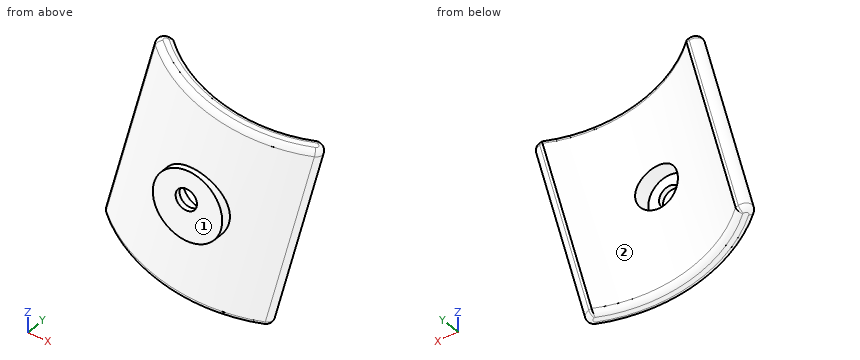
from build123d import *

# Parameters (mm, degrees)
CYLINDER016_R          = 8
CYLINDER016_DEPTH      = 10
CYLINDER016_ROLL_ANGLE = 90
CYLINDER015_R          = 4
CYLINDER015_DEPTH      = 20
CYLINDER015_ROLL_ANGLE = 90
BOX016_W               = 120
BOX016_H               = 100
BOX016_DEPTH           = 150
CYLINDER014_R          = 44
CYLINDER014_DEPTH      = 75
CYLINDER013_R          = 50
CYLINDER013_DEPTH      = 75
CYLINDER012_R          = 13
CYLINDER012_DEPTH      = 8
CYLINDER012_ROLL_ANGLE = 90
FILLET012_R            = 3
FILLET013_R            = 2
FILLET014_R            = 2
CUT021_PITCH_ANGLE     = 15


with BuildPart() as cylindre016:
    # Cylinder016 → Cylinder016 (new body)
    with BuildSketch(Plane.XY):
        Circle(CYLINDER016_R)
    extrude(amount=CYLINDER016_DEPTH)


with BuildPart() as cylindre016_1:
    # Cylinder016 roll: moved
    add(cylindre016.part.rotate(Axis((0, 0, 0), (1, 0, 0)), CYLINDER016_ROLL_ANGLE))


with BuildPart() as cylindre016_2:
    # Cylinder016 placement: moved
    add(cylindre016_1.part.moved(Location((-212, -9, -164))))


with BuildPart() as cylindre015:
    # Cylinder015 → Cylinder015 (new body)
    with BuildSketch(Plane.XY):
        Circle(CYLINDER015_R)
    extrude(amount=CYLINDER015_DEPTH)


with BuildPart() as cylindre015_1:
    # Cylinder015 roll: moved
    add(cylindre015.part.rotate(Axis((0, 0, 0), (1, 0, 0)), CYLINDER015_ROLL_ANGLE))


with BuildPart() as cylindre015_2:
    # Cylinder015 placement: moved
    add(cylindre015_1.part.moved(Location((-212, -10, -164))))


with BuildPart() as cube016:
    # Box016 → Box016 (new body)
    with BuildSketch(Plane(origin=(-269, -3, -220), x_dir=(1, 0, 0), z_dir=(0, 0, 1))):
        with Locations((60, 50)):
            Rectangle(BOX016_W, BOX016_H)
    extrude(amount=BOX016_DEPTH)


with BuildPart() as cylindre014:
    # Cylinder014 → Cylinder014 (new body)
    with BuildSketch(Plane(origin=(-212, 31, -203), x_dir=(1, 0, 0), z_dir=(0, 0, 1))):
        Circle(CYLINDER014_R)
    extrude(amount=CYLINDER014_DEPTH)


with BuildPart() as cut017:
    # Cylinder013 → Cylinder013 (new body)
    with BuildSketch(Plane(origin=(-212, 31, -203), x_dir=(1, 0, 0), z_dir=(0, 0, 1))):
        Circle(CYLINDER013_R)
    extrude(amount=CYLINDER013_DEPTH)

    # Cut017: cut Cylindre014
    add(cylindre014.part, mode=Mode.SUBTRACT)


with BuildPart() as cut021:
    # Cylinder012 → Cylinder012 (new body)
    with BuildSketch(Plane.XY):
        Circle(CYLINDER012_R)
    extrude(amount=CYLINDER012_DEPTH)


with BuildPart() as cut021_1:
    # Cylinder012 roll: moved
    add(cut021.part.rotate(Axis((0, 0, 0), (1, 0, 0)), CYLINDER012_ROLL_ANGLE))


with BuildPart() as cut021_2:
    # Cylinder012 placement: moved
    add(cut021_1.part.moved(Location((-211, -13, -166))))

    # Fusion011: union Cut017
    add(cut017.part)

    # Cut018: cut Cube016
    add(cube016.part, mode=Mode.SUBTRACT)

    # Fillet012
    fillet012_edges = [cut021_2.edges().sort_by_distance(p)[0] for p in [
        (-175.339394, -3, -165.5),
        (-248.660606, -3, -165.5),
    ]]
    fillet(fillet012_edges, radius=FILLET012_R)

    # Fillet013
    fillet013_edges = [cut021_2.edges().sort_by_distance(p)[0] for p in [
        (-212, -19, -203),
        (-212, -13, -203),
    ]]
    fillet(fillet013_edges, radius=FILLET013_R)

    # Fillet014
    fillet014_edges = [cut021_2.edges().sort_by_distance(p)[0] for p in [
        (-212, -19, -128),
        (-212, -13, -128),
    ]]
    fillet(fillet014_edges, radius=FILLET014_R)

    # Cut019: cut Cylindre015
    add(cylindre015_2.part, mode=Mode.SUBTRACT)

    # Cut021: cut Cylindre016
    add(cylindre016_2.part, mode=Mode.SUBTRACT)


with BuildPart() as cut021_3:
    # Cut021 pitch: moved
    add(cut021_2.part.rotate(Axis((0, 0, 0), (0, 1, 0)), CUT021_PITCH_ANGLE))


with BuildPart() as cut021_4:
    # Cut021 placement: moved
    add(cut021_3.part.moved(Location((35.610827, 0, -60.508913))))


solid = cut021_4.part
Can you work these out from the model? Positions are in its coordinate system, mm. Face numbers are marked on the shaded views. Give positions to 0.01 mm unless a question says otherwise; leave off trailing zeros. One line per item, written item: value.
1) I'm going to push flat-ended pins straight in: pin 1 (4 mm diameter, centred on y = -9, z = -163, fed in from +X); pin 2 (2 mm diameter, centred on x = -193.5, z = -190.5, fed in from +Y); pin 3 (4 mm diameter, centred on x = -232, y = -13, fed in from -Z). Where does each tip first touch, or does it pass through?
Geometry check:
pin 1: stops at x = -178.24
pin 2: stops at y = -4.97
pin 3: stops at z = -199.43
2) Thinking about a two-plate mould opening in X: for the marked faces 1 and 2, which applies, +X half, -X half, draft (parallel to the pull), parting line (faces both ways), or undercut?
Geometry check:
face 1: draft
face 2: undercut
3) Please list where these lines run through material, in increasing order: line 1 (Z direction, x = -217.5, y = -15.5); line 2 (X direction, y = -9, z = -190); line 3 (X direction, y = -5.5, z = -172).
Geometry check:
line 1: z = -202.85 to -169.47, -158.64 to -125.52
line 2: x = -249.62 to -237.54, -199.59 to -187.51
line 3: x = -246.81 to -239.18, -188.3 to -180.67
